Design review of the part built by this model. Coordinates are the model's own, in mm. Give positions to 0.01 mm unless a question says otherwise; leave off trailing zeros. Loops run counter-clockwise (first coordinate to the right, second up) from the corner with the lowest first, then second, coordinate; pieces in that order, holes last. Notation, with made-up numbers: M 0,64.5 L 5,64.5 A28 ccw 5,95.5 Z; hole C -11,35.25 d3. An arc over 180 degrees is marked long. Use one line per item in the form item = value. Start each with the question number.
from build123d import *

# Parameters (mm, degrees)
CROQUIS1_R              = 60
SALIENTE_EXTRUIR1_DEPTH = 4.7625
CROQUIS2_R              = 3.25
CORTAR_EXTRUIR1_DEPTH   = 85.986360119
CHAFL_N1_SIZE           = 1.5
CROQUIS3_R              = 11
CORTAR_EXTRUIR2_DEPTH   = 85.986360119
CROQUIS4_R              = 3.25
CORTAR_EXTRUIR3_DEPTH   = 85.986360119
CHAFL_N2_SIZE           = 0.5
CHAFL_N3_SIZE           = 3


with BuildPart() as part:
    # Croquis1 → Saliente-Extruir1 (new body)
    with BuildSketch(Plane.XY):
        with Locations(Location((0, 0, 0), (0, 0, 180))):
            Circle(CROQUIS1_R)
    extrude(amount=SALIENTE_EXTRUIR1_DEPTH)

    # Croquis2 → Cortar-Extruir1 (cut, through all)
    with BuildSketch(Plane.XY.offset(4.7625)):
        with Locations((50, 0)):
            Circle(CROQUIS2_R)
        with Locations((35.355339059, -35.355339059)):
            Circle(CROQUIS2_R)
        with Locations((0, -50)):
            Circle(CROQUIS2_R)
        with Locations((-35.355339059, -35.355339059)):
            Circle(CROQUIS2_R)
        with Locations((-50, 0)):
            Circle(CROQUIS2_R)
        with Locations((-35.355339059, 35.355339059)):
            Circle(CROQUIS2_R)
        with Locations((0, 50)):
            Circle(CROQUIS2_R)
        with Locations((35.355339059, 35.355339059)):
            Circle(CROQUIS2_R)
    extrude(amount=-CORTAR_EXTRUIR1_DEPTH, mode=Mode.SUBTRACT)

    # Chaflán1
    chafl_n1_edges = [part.edges().sort_by_distance(p)[0] for p in [
        (60, 0, 4.7625),
    ]]
    chamfer(chafl_n1_edges, length=CHAFL_N1_SIZE)

    # Croquis3 → Cortar-Extruir2 (cut, through all)
    with BuildSketch(Plane.XY.offset(4.7625)):
        Circle(CROQUIS3_R)
    extrude(amount=-CORTAR_EXTRUIR2_DEPTH, mode=Mode.SUBTRACT)

    # Croquis4 → Cortar-Extruir3 (cut, through all)
    with BuildSketch(Plane.XY.offset(4.7625)):
        with Locations((20, 20)):
            Circle(CROQUIS4_R)
        with Locations((-20, 20)):
            Circle(CROQUIS4_R)
        with Locations((-20, -20)):
            Circle(CROQUIS4_R)
        with Locations((20, -20)):
            Circle(CROQUIS4_R)
    extrude(amount=-CORTAR_EXTRUIR3_DEPTH, mode=Mode.SUBTRACT)

    # Chaflán2
    chafl_n2_edges = [part.edges().sort_by_distance(p)[0] for p in [
        (32.105339059, -35.355339059, 4.7625),
        (-3.25, -50, 4.7625),
        (-38.605339059, -35.355339059, 4.7625),
        (-53.25, 0, 4.7625),
        (-38.605339059, 35.355339059, 4.7625),
        (-3.25, 50, 4.7625),
        (32.105339059, 35.355339059, 4.7625),
        (-11, 0, 0),
        (-11, 0, 4.7625),
        (46.75, 0, 4.7625),
    ]]
    chamfer(chafl_n2_edges, length=CHAFL_N2_SIZE)

    # Chaflán3
    chafl_n3_edges = [part.edges().sort_by_distance(p)[0] for p in [
        (16.75, 20, 4.7625),
        (-23.25, 20, 4.7625),
        (-23.25, -20, 4.7625),
        (16.75, -20, 4.7625),
    ]]
    chamfer(chafl_n3_edges, length=CHAFL_N3_SIZE)


solid = part.part
Q1. Take a section at B-B on z = 2.5. State how many separate pieces and enclosed holes the cut face has, plus the area to 3 significant figures.
Q2. The part is to be moulded in two halves that separate along X. For faces 1 (the cylindrical face through (-32.26, -50.59, 1.61)), 2 (the cylindrical face through (17.605, -17.803, 0.894)), 3 (the flat face through (-12, -1, 0)), say which applies: pulls with the +X half, pulls with the -X half, needs draft (parallel to the pull), parting line crosses it, or undercut.
Q3. Take a section at A-A on x = 0. Give the boundary of the cut face in (y, z), plus the area to 3 significant figures.
Q4. Clearance check with flat-ended pins moving along their axes: pin 1 Ø4 at (x, y) = (-35.36, 35.36) entering from -Z; pin 2 Ø10.5 at (x, y) = (20, -20) entering from +Z; pin 3 Ø2 at (y, z) = (40, 1) entering from -X; pin 4 Ø2 at (x, z) = (-27.5, 1) entering from +Y. State where each tip first meets the part, or that it passes through.
Q5. Wall thickness on probe 1 along X at (y, z) = (1.5, 0.7); probe 2 along Y at (x, z) = (-20, 0.7); probe 3 along Y at (x, z) = (0.5, 2.55): over which ranges is each line inside the solid? List them lowest first.
Response values:
q1.separate_pieces = 1
q1.enclosed_holes = 13
q1.area = 10,500 mm^2
q2.face_1 = parting line crosses it
q2.face_2 = undercut
q2.face_3 = needs draft
q3.outline = M -60,0 L -53.25,0 L -53.25,4.26 L -53.75,4.76 L -58.5,4.76 L -60,3.26 Z; M -46.75,0 L -11.5,0 L -11,0.5 L -11,4.26 L -11.5,4.76 L -46.25,4.76 L -46.75,4.26 Z; M 11,0.5 L 11.5,0 L 46.75,0 L 46.75,4.26 L 46.25,4.76 L 11.5,4.76 L 11,4.26 Z; M 53.25,0 L 60,0 L 60,3.26 L 58.5,4.76 L 53.75,4.76 L 53.25,4.26 Z
q3.area = 402 mm^2
q4.pin_1 = through
q4.pin_2 = 3.76
q4.pin_3 = -45.6
q4.pin_4 = 53.83
q5.probe_1 = -59.98 to -52.88, -47.12 to -10.9, 10.9 to 47.12, 52.88 to 59.98
q5.probe_2 = -56.57 to -23.25, -16.75 to 16.75, 23.25 to 56.57
q5.probe_3 = -60 to -53.21, -46.79 to -10.99, 10.99 to 46.79, 53.21 to 60
